Input: part model. Units: mm. Frame: model coordinates. Face numbers are marked on the shaded views. A direction names the side the tool comes from. Give positions to 0.01 mm unless a question says otherwise; leave off trailing zeros. Loops run counter-clockwise (first coordinate to the right, second up) from the corner with the lowest first, then second, coordinate; pieces in that order, holes last. Notation, with made-up numbers: (52.5, -2.75) - (101.5, -2.75) arc R23 ccw to (101.5, 20.25) - close; hole circle Ø4 at (60.5, 20). An arc over 180 degrees is marked (long way). One line per item, written item: value.
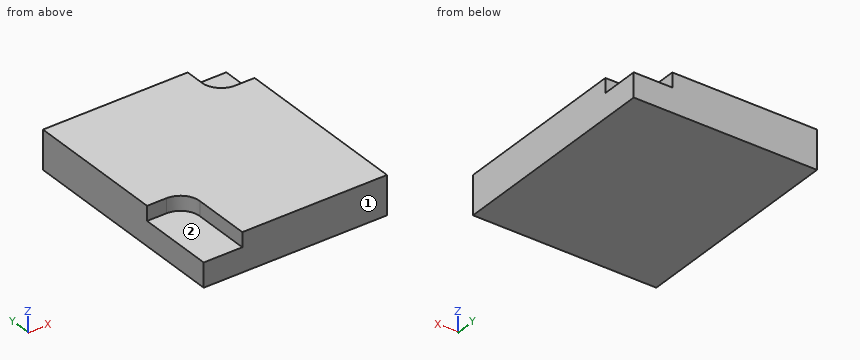
from build123d import *

# Parameters (mm, degrees)
SKETCH001_W     = 9.5
SKETCH001_H     = 11.35
PAD002_DEPTH    = 2
POCKET_DEPTH    = 0.75
POCKET001_DEPTH = 0.75


with BuildPart() as part:
    # Sketch001 → Pad002 (new body)
    with BuildSketch(Plane.XY.offset(5.5)):
        with Locations((0, -0.825)):
            Rectangle(SKETCH001_W, SKETCH001_H)
    extrude(amount=PAD002_DEPTH)

    # Sketch003 → Pocket (cut)
    with BuildSketch(Plane.XY.offset(7.5)):
        with BuildLine():
            Line((2.75, 4.85), (4.75, 4.85))
            Line((4.75, 4.85), (4.75, 2.85))
            Line((4.75, 2.85), (3.75, 2.85))
            ThreePointArc((2.75, 3.85), (3.042893, 3.142893), (3.75, 2.85))
            Line((2.75, 3.85), (2.75, 4.85))
        make_face()
    extrude(amount=-POCKET_DEPTH, mode=Mode.SUBTRACT)

    # Sketch004 → Pocket001 (cut)
    with BuildSketch(Plane.XY.offset(7.5)):
        with BuildLine():
            Line((-4.75, -2.5), (-3.75, -2.5))
            ThreePointArc((-2.75, -3.5), (-3.042893, -2.792893), (-3.75, -2.5))
            Line((-2.75, -3.5), (-2.75, -6.5))
            Line((-2.75, -6.5), (-4.75, -6.5))
            Line((-4.75, -6.5), (-4.75, -2.5))
        make_face()
    extrude(amount=-POCKET001_DEPTH, mode=Mode.SUBTRACT)


solid = part.part
Item 1: Material intervals for L1, parallel to Y at x = 4.5, z = 7.05; L2, parallel to Z at x = 3.5, y = 3; L3, parallel to X at y = 3, z = 7.2, sorted ascending.
Verdict:
L1: y = -6.5 to 2.85
L2: z = 5.5 to 6.75
L3: x = -4.75 to 3.22
Item 2: Section B-B, the plane z = 7.3. Output: boundary loops of the cut face in (x, y).
Verdict:
outline: (-4.75, -2.5) - (-3.75, -2.5) arc R1 cw to (-2.75, -3.5) - (-2.75, -6.5) - (4.75, -6.5) - (4.75, 2.85) - (3.75, 2.85) arc R1 cw to (2.75, 3.85) - (2.75, 4.85) - (-4.75, 4.85) - close
Item 3: Pin query (flat end, axial travel): P1, Ø2, axis at x = 4, y = 4, coming from the +Z side. Return the tip coordinate at first contact, or that it passes through.
Verdict:
P1: stops at z = 6.75
Item 4: Access query for the marked faces 1 and 2. Directions: +Z, -Z, +X, -X, +Y, -Y. A direction counts if a zero-diameter tool reaches every point of the face in a straight line with its end or side. Return the directions, or none.
Verdict:
face 1: +Z, -Z, +X, -X, -Y
face 2: +Z, -X, -Y
Item 5: Section C-C, the plane y = 3.25. Output: boundary loops of the cut face in (x, z).
Verdict:
outline: (-4.75, 5.5) - (4.75, 5.5) - (4.75, 6.75) - (2.95, 6.75) - (2.95, 7.5) - (-4.75, 7.5) - close
Item 6: Section A-A, the plane x = 4. Output: boundary loops of the cut face in (y, z), and give its area (3 significant figures).
Verdict:
outline: (-6.5, 5.5) - (4.85, 5.5) - (4.85, 6.75) - (2.85, 6.75) - (2.85, 7.5) - (-6.5, 7.5) - close
area: 21.2 mm^2
